```python
from build123d import *

# Parameters (mm, degrees)
SKICA1_W                 = 55.6
SKICA1_H                 = 55.6
P_IDAT_VYSUNUT_M2_DEPTH  = 3
SKICA5_W                 = 55.6
SKICA5_H                 = 5
ODEBRAT_VYSUNUT_M3_DEPTH = 1
SKICA14_W                = 53.6
SKICA14_H                = 1.5
P_IDAT_VYSUNUT_M9_DEPTH  = 9.5
SKICA17_R                = 2
ODEBRAT_VYSUNUT_M8_DEPTH = 4
SKICA19_W                = 6.8
SKICA19_H                = 6.8
P_IDAT_VYSUNUT_M10_DEPTH = 12.5
SKICA20_R                = 2.4
ODEBRAT_VYSUNUT_M9_DEPTH = 1.7
ZAOBLIT1_R               = 2.5


with BuildPart() as part:
    # Skica1 → Přidat vysunutím2 (new body)
    with BuildSketch(Plane.XY):
        Rectangle(SKICA1_W, SKICA1_H)
    extrude(amount=P_IDAT_VYSUNUT_M2_DEPTH)

    # Skica5 → Odebrat vysunutím3 (cut)
    with BuildSketch(Plane(origin=(0, 0, 0), x_dir=(-1, 0, 0), z_dir=(0, 0, -1))):
        Rectangle(SKICA5_W, SKICA5_H)
    extrude(amount=-ODEBRAT_VYSUNUT_M3_DEPTH, mode=Mode.SUBTRACT)

    # Skica14 → Přidat vysunutím9 (add)
    with BuildSketch(Plane.XY.offset(3)):
        Polygon((27.8, 27.8), (-27.8, 27.8), (-27.8, -27.8), (-26.8, -27.8), (-26.8, -26.8), (-26.8, -26.3), (-26.8, 26.8), (26.8, 26.8), (26.8, -26.3), (26.8, -27.8), (27.8, -27.8), align=None)
        with Locations((0, -27.05)):
            Rectangle(SKICA14_W, SKICA14_H)
    extrude(amount=P_IDAT_VYSUNUT_M9_DEPTH)

    # Skica17 → Odebrat vysunutím8 (cut)
    with BuildSketch(Plane(origin=(0, 0, 1), x_dir=(-1, 0, 0), z_dir=(0, 0, -1))):
        with Locations((-20.8, 0)):
            Circle(SKICA17_R)
        with Locations((20.8, 0)):
            Circle(SKICA17_R)
    extrude(amount=-ODEBRAT_VYSUNUT_M8_DEPTH, mode=Mode.SUBTRACT)

    # Skica19 → Přidat vysunutím10 (add)
    with BuildSketch(Plane(origin=(0, 0, 0), x_dir=(-1, 0, 0), z_dir=(0, 0, -1))):
        with Locations((-24.4, 24.4)):
            Rectangle(SKICA19_W, SKICA19_H)
        with Locations((24.4, 24.4)):
            Rectangle(SKICA19_W, SKICA19_H)
        with Locations((-24.4, -24.4)):
            Rectangle(SKICA19_W, SKICA19_H)
        with Locations((24.4, -24.4)):
            Rectangle(SKICA19_W, SKICA19_H)
    extrude(amount=-P_IDAT_VYSUNUT_M10_DEPTH)

    # Skica20 → Odebrat vysunutím9 (cut)
    with BuildSketch(Plane.XY.offset(12.5)):
        with Locations((-23.9, -23.9)):
            Circle(SKICA20_R)
        with Locations((-23.9, 23.9)):
            Circle(SKICA20_R)
        with Locations((23.900280565, 23.9)):
            Circle(SKICA20_R)
        with Locations((23.900280565, -23.9)):
            Circle(SKICA20_R)
    extrude(amount=-ODEBRAT_VYSUNUT_M9_DEPTH, mode=Mode.SUBTRACT)

    # Zaoblit1
    zaoblit1_edges = [part.edges().sort_by_distance(p)[0] for p in [
        (21, -21, 7.75),
        (-21, -21, 7.75),
        (21, 21, 7.75),
        (-21, 21, 7.75),
    ]]
    fillet(zaoblit1_edges, radius=ZAOBLIT1_R)


solid = part.part
```
Can you work these out from the model? Positions are in its coordinate system, mm. A direction names the side the tool comes from. Coordinates: 2 decimals unless noted, no trailing zeros. Loops run counter-clockwise (first coordinate to the right, second up) from the corner with the lowest first, then second, coordinate; pieces in that order, holes last. Notation, with made-up numbers: (46.25, 13.5) -> (76.25, 13.5) arc R21 ccw to (76.25, 37.5) -> close; hole circle Ø10 at (18, 33). An arc over 180 degrees is marked (long way). Put each result on its own line as item: value. Start each with the question number.
Q1. I want a section at B-B (z = 7.75). Write out the boundary of the cut face in (x, y).
Q2. I want a section at C-C (x = -15). Write out the boundary of the cut face in (y, z).
Q3. Thinking about a two-plate mould opening in X: for faces 3 (the face through (0, -27.8, 6)), 4 (the face through (25.191, -21.876, 11.662)), which applies, pulls with the +X half, pulls with the -X half, needs draft (parallel to the pull), parting line crosses it, or undercut?
Q4. For faces 1 (the face through (0, 27.8, 6)), 2 (the face through (21, -25, 8)), which set-ups out of +Z, -Z, +X, -X, +Y, -Y let a thin tool reach every point of the face, with its end or its side?
Q5. If I drill on line 1 (Y direction, x = -23.9, z = 11.8); line 2 (Y direction, x = -20.8, z = 2.1); line 3 (Y direction, x = -5.5, z = 5.5), over which ranges is the centre line in solid material (lowest first)? Write a range as [from, to].
Q6. I'm going to push flat-ended pins straight in: P1, Ø3, axis at x = 23.9, y = 23.9, coming from the +Z side; P2, Ø12, axis at x = 8, y = 2, coming from the +Z side. Where does each tip first touch, or does it pass through?
Q7. I want a section at A-A (y = 0). Write out the boundary of the cut face in (x, z), plus the area to 3 significant figures.
Taken from the geometry:
1. outline: (-27.8, -27.8) -> (27.8, -27.8) -> (27.8, 27.8) -> (-27.8, 27.8) -> close; hole (-26.8, -21) -> (-23.5, -21) arc R2.5 cw to (-21, -23.5) -> (-21, -26.3) -> (21, -26.3) -> (21, -23.5) arc R2.5 cw to (23.5, -21) -> (26.8, -21) -> (26.8, 21) -> (23.5, 21) arc R2.5 cw to (21, 23.5) -> (21, 26.8) -> (-21, 26.8) -> (-21, 23.5) arc R2.5 cw to (-23.5, 21) -> (-26.8, 21) -> close
2. outline: (-27.8, 0) -> (-2.5, 0) -> (-2.5, 1) -> (2.5, 1) -> (2.5, 0) -> (27.8, 0) -> (27.8, 12.5) -> (26.8, 12.5) -> (26.8, 3) -> (-26.3, 3) -> (-26.3, 12.5) -> (-27.8, 12.5) -> close
3. face 3: needs draft
3. face 4: undercut
4. face 1: +Z, -Z, +X, -X, +Y
4. face 2: +Z
5. line 1: y = [-27.8, -26.3], [-21.5, -21], [21, 21.5], [26.3, 27.8]
5. line 2: y = [-27.8, -2], [2, 27.8]
5. line 3: y = [-27.8, -26.3], [26.8, 27.8]
6. P1: stops at z = 10.8
6. P2: stops at z = 3
7. outline: (-27.8, 1) -> (-22.8, 1) -> (-22.8, 3) -> (-26.8, 3) -> (-26.8, 12.5) -> (-27.8, 12.5) -> close; (-18.8, 1) -> (18.8, 1) -> (18.8, 3) -> (-18.8, 3) -> close; (22.8, 1) -> (27.8, 1) -> (27.8, 12.5) -> (26.8, 12.5) -> (26.8, 3) -> (22.8, 3) -> close
7. area: 114 mm2
